from build123d import *

# Parameters (mm, degrees)
F0_R     = 4.05
F1_DEPTH = 6
F0_R_2   = 5
F2_DEPTH = 2.5
F0_R_3   = 10
F3_DEPTH = 2
F4_R     = 1


with BuildPart() as f1:
    # F0 (on Top) → F1 (new body)
    with BuildSketch(Plane.XY):
        Circle(F0_R)
    extrude(amount=-F1_DEPTH)

    # F0 (on Top) → F2 (join)
    with BuildSketch(Plane.XY):
        Circle(F0_R_2)
        Circle(F0_R, mode=Mode.SUBTRACT)
    extrude(amount=-F2_DEPTH)

    # F0 (on Top) → F3 (join)
    with BuildSketch(Plane.XY):
        Circle(F0_R_3)
        Circle(F0_R_2, mode=Mode.SUBTRACT)
    extrude(amount=-F3_DEPTH)

    # F4
    f4_edges = [f1.edges().sort_by_distance(p)[0] for p in [
        (-10, 0, 0),
    ]]
    fillet(f4_edges, radius=F4_R)


solid = f1.part
The listing builds one solid part. Answer for the finished solid, in the listing's coordinates (mm). A direction names the side the tool comes from. Give positions to 0.01 mm unless a question says otherwise; leave off trailing zeros. Order: outer loops, then holes, each group sorted by start corner. A loop starts at its lowest first (then second) coordinate and runs counter-clockwise, first axis right, second up. Notation, with made-up numbers: (-29.5, -36) - (9.5, -36) arc R20 cw to (9.5, -7) - close; hole circle Ø4 at (-22, 72). An arc over 180 degrees is marked (long way). Answer as CSV lines item,"result".
Q1. A cutting plane is placed at C-C, the plane z = -4.2. Determine the outline of the cut face in (x, y).
Answer key:
outline,"circle Ø8.1 at (0, 0)"
Q2. Which of the six approach directions +Z, -Z, +X, -X, +Y, -Y give full straight-line access (tool end or side, diameter ignored) to faces 1 (the face through (-5, -2, -2)), 2 (the face through (0, 0, -6))?
Answer key:
face 1,"-Z"
face 2,"-Z, +X, -X, +Y, -Y"
Q3. Each of these flat-tipped pins is pushed along its axis until it touches: pin 1 Ø3 at (y, z) = (6.5, -2.5) entering from -X; pin 2 Ø1 at (y, z) = (-2.5, -1) entering from +X; pin 3 Ø2 at (x, z) = (6.5, -2) entering from +Y; pin 4 Ø6 at (x, y) = (-2.5, 4.5) entering from -Z. Where does it stop, or does it pass through?
Answer key:
pin 1,"stops at x = -8.61"
pin 2,"stops at x = 9.8"
pin 3,"stops at y = 8.35"
pin 4,"stops at z = -6"
Q4. A cutting plane is placed at A-A, the plane y = 0. Determine the outline of the cut face in (x, z), and give its area (3 significant figures).
Answer key:
outline,"(-10, -2) - (-5, -2) - (-5, -2.5) - (-4.05, -2.5) - (-4.05, -6) - (4.05, -6) - (4.05, -2.5) - (5, -2.5) - (5, -2) - (10, -2) - (10, -1) arc R1 ccw to (9, 0) - (-9, 0) arc R1 ccw to (-10, -1) - close"
area,"72.9 mm^2"
Q5. Straight lines are drawn through the part: L1, parallel to Z at x = -5, y = 7; L2, parallel to Z at x = -3.25, y = -2.75; L3, parallel to Y at x = 2.5, z = -5.3. For each, find the intervals that lie inside material, in ascending order.
Answer key:
L1,"z = -2 to 0"
L2,"z = -2.5 to 0"
L3,"y = -3.19 to 3.19"
